Autodesk Inventor part; units mm, degrees
ref_plane "YZ Plane" through (0, 0, 0) normal (1, 0, 0) x (0, 1, 0)
ref_plane "XZ Plane" through (0, 0, 0) normal (0, 1, 0) x (-1, 0, 0)
ref_plane "XY Plane" through (0, 0, 0) normal (0, 0, 1) x (1, 0, 0)
sketch "Sketch1" plane through (0, 0, 0) normal (0, 0, 1) x (1, 0, 0)
  circle A0 centre (0, 0) radius 7
  dimension "d0" = 14
extrude "Extrusion1" add sketch "Sketch1" along normal blind 5
sketch "Sketch2" plane through (0, 0, 5) normal (0, 0, 1) x (1, 0, 0)
  point P0 (0, 0)
  point P1 (0, 0)
hole "Hole1" at (0, 0, 5) direction (0, 0, -1) diameter 4.5 end through all countersink diameter 9.4 countersink angle 90
chamfer "Chamfer1" distance 0.5 angle 45 1 edges at (-7, 0, 0)
properties part number "Top_Lever End Piece" material "Stainless Steel"
The model under review builds one solid part; all positions refer to its coordinate system, in mm. Round coordinates to 2 decimals unless told otherwise and drop trailing zeros. Write each loop counter-clockwise with the first axis right and the second up, starting at its lowest first coordinate (ties: lowest second). Pieces come first, ordered by that corner, then holes. Notation, with made-up numbers: (31.5, -21.5) - (79.5, -21.5) arc R15 cw to (79.5, -0.5) - close; hole circle Ø7 at (59, -32.5). An arc over 180 degrees is marked (long way). One line per item, written item: value. Start each with the question number.
1. Clearance check with flat-ended pins moving along their axes: P1, Ø3, axis at x = -3.5, y = 1.5, coming from the -Z side; P2, Ø1, axis at x = -5, z = 2.5, coming from the -Y side; P3, Ø1.5, axis at y = 4.5, z = 3.5, coming from the +X side; P4, Ø1.5, axis at y = -1, z = 1, coming from the -X side. State where each tip first meets the part, or that it passes through.
2. To check wall thickness, follow L1, parallel to Y at x = 0, z = 0.65; L2, parallel to Y at x = 1, z = 0.65; L3, parallel to X at y = -2.25, z = 3.4. State the ranges of each line that lie inside material, in increasing order. Write a range as from..to.
3. Consider section C-C on z = 1.1. Write out the cut boundary in (x, y).
4. Consider section A-A on x = 0. Write out the cut boundary in (y, z), and give its area (3 significant figures).
5. The part is to be moulded in two halves that separate along X. For faces 1 (the face through (-2.23, 0.29, 1.26)), 2 (the face through (6.466, 2.681, 2.718)), 3 (the face through (3, 0, 0)), say which applies: released by +X, released by -X, zero draft, split by the parting line, or undercut.
Checks:
1. P1: stops at z = 0
1. P2: stops at y = -5.36
1. P3: stops at x = 5.91
1. P4: stops at x = -7
2. L1: y = -7..-2.25, 2.25..7
2. L2: y = -6.93..-2.02, 2.02..6.93
2. L3: x = -6.63..-2.13, 2.13..6.63
3. outline: circle Ø14 at (0, 0); hole circle Ø4.5 at (0, 0)
4. outline: (-7, 0.5) - (-6.5, 0) - (-2.25, 0) - (-2.25, 2.55) - (-4.7, 5) - (-7, 5) - close; (2.25, 0) - (6.5, 0) - (7, 0.5) - (7, 5) - (4.7, 5) - (2.25, 2.55) - close
4. area: 41.2 mm^2
5. face 1: undercut
5. face 2: split by the parting line
5. face 3: zero draft
